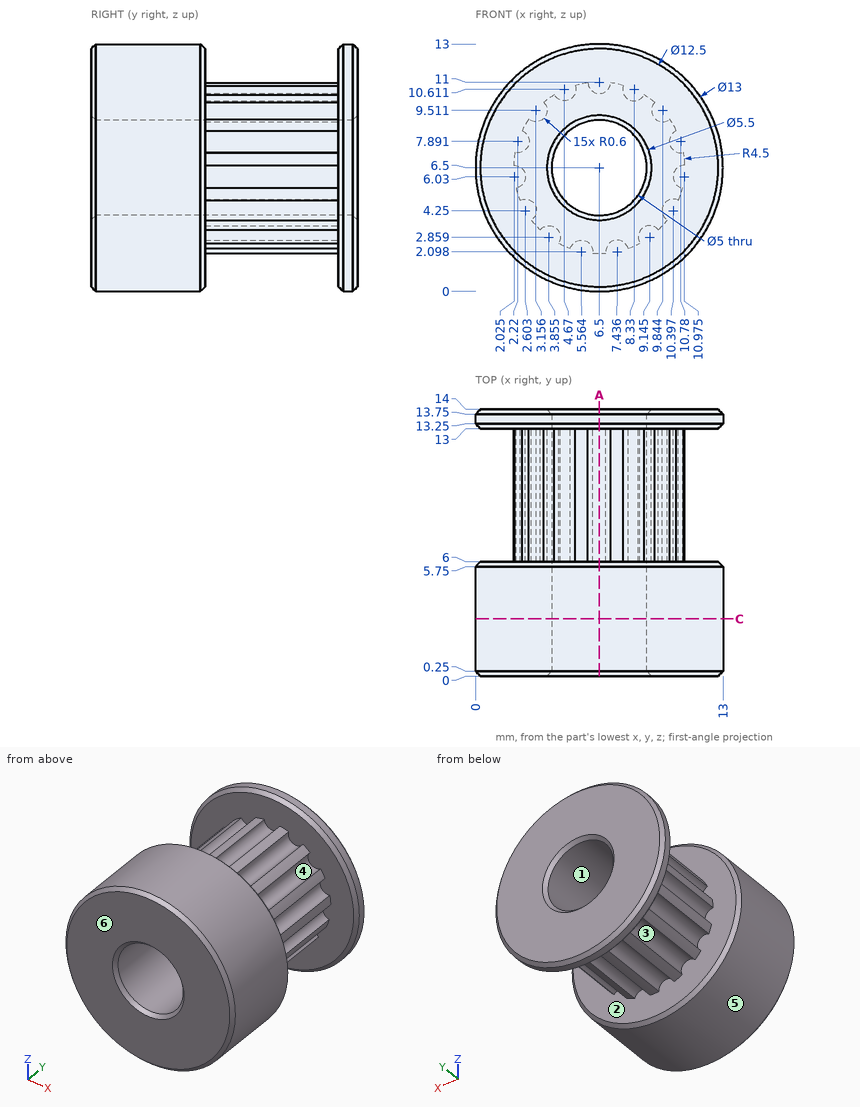
Design review of the part shown in the three views and the two pictorial views. Dimensions are in mm from the part's minimum x, y and z. A direction names the side the tool comes from. Give positions to 0.01 mm unless a question says otherwise; leave off trailing zeros. Write each loop counter-clockwise with the first axis right and the second up, starting at its lowest first coordinate (ties: lowest second). Pieces come first, ordered by that corner, then holes.
(1) Clearance check with flat-ended pins moving along their axes: pin 1 Ø1 at (x, y) = (10, 12) entering from +Z; pin 2 Ø1 at (y, z) = (10, 11) entering from +X. State where each tip first meets the part, or that it passes through.
Checked values:
pin 1: stops at z = 9.04
pin 2: stops at x = 7.77
(2) Mouldability with a two-part tool opening along X and no side actions: class the marked faces 3, 4, 5 and 6 as +X half, -X half, draft (parallel to the pull), parting line (faces both ways), or undercut.
Checked values:
face 3: undercut
face 4: undercut
face 5: parting line
face 6: draft
(3) Wall thickness on line 1 along Z through (x, y) = (6.5, 3); line 2 along Y through (x, z) = (3.25, 3); line 3 along Z through (x, y) = (6.5, 6.75): over which ranges is each line inside the solid? List them lowest first.
Checked values:
line 1: z = 0 to 4, 9 to 13
line 2: y = 0 to 6, 13 to 14
line 3: z = 2 to 4, 9 to 10.4
(4) Add section A-A (x = 6.5). Give the boundary of the cut face in (y, z).
Checked values:
outline: (0, 0.25) - (0.25, 0) - (5.75, 0) - (6, 0.25) - (6, 2) - (13, 2) - (13, 0.25) - (13.25, 0) - (13.75, 0) - (14, 0.25) - (14, 3.75) - (13.75, 4) - (0.25, 4) - (0, 3.75) - close; (0, 9.25) - (0.25, 9) - (13.75, 9) - (14, 9.25) - (14, 12.75) - (13.75, 13) - (13.25, 13) - (13, 12.75) - (13, 10.4) - (6, 10.4) - (6, 12.75) - (5.75, 13) - (0.25, 13) - (0, 12.75) - close
(5) Tool access review of the marked faces 1 and 2: name each direction out of +Z, -Z, +X, -X, +Y, -Y from which nothing blocks a thin tool from reaching the whole face with its end or side.
Checked values:
face 1: +Y, -Y
face 2: none
(6) Add section C-C (y = 3). Give the boundary of the cut face in (x, z).
Checked values:
outline: circle Ø13 at (6.5, 6.5); hole circle Ø5 at (6.5, 6.5)
